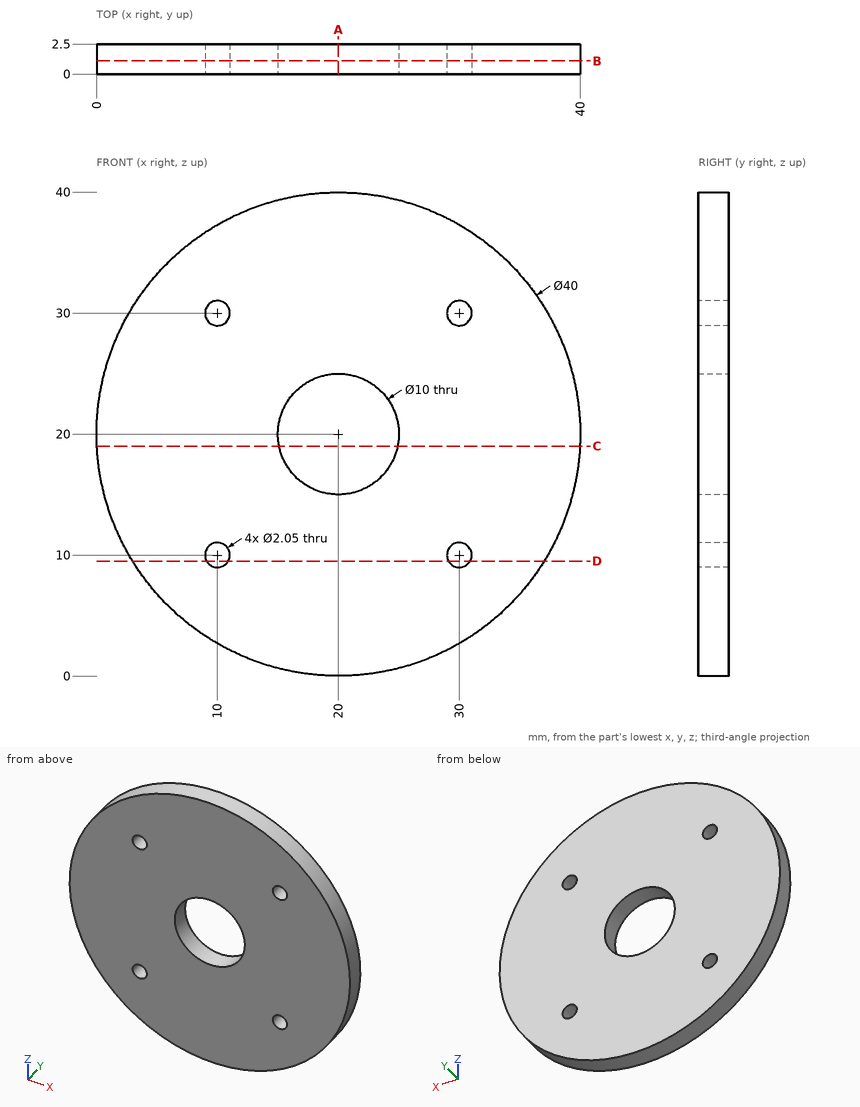
Input: dimensioned drawing with shaded views. Units: mm. Origin: part minimum x, y, z. Coordinates: 2 decimals unless noted, no trailing zeros. Loops run counter-clockwise (first coordinate to the right, second up) from the corner with the lowest first, then second, coordinate; pieces in that order, holes last. Notation, with made-up numbers: (18, 40) -> (65, 40) arc R35 ccw to (65, 79) -> close; hole circle Ø1 at (48.25, -21). An arc over 180 degrees is marked (long way). One line per item, written item: value. Start each with the question number.
Q1. Section query A-A, the plane x = 20. Return the cut outline in (y, z).
Q2. Section query C-C, the plane z = 19. Return the cut outline in (x, y).
Q3. Section query B-B, the plane y = 1.1. Return the cut outline in (x, z) (3 decimals), and give its area (3 significant figures).
Q4. Line query: line 1 along X through (y, z) = (1.85, 10) (1 decimal); line 2 along Z through (x, y) = (17.5, 1.75). Output: solid intervals per line, ascending.
Q5. Contact query for flat-ended pins moving along their axis: P1, Ø2.5, axis at x = 10, z = 10, coming from the -Y side; P2, Ø9, axis at x = 20, z = 20, coming from the +Y side; P3, Ø1, axis at y = 0.5, z = 31, coming from the +X side; P4, Ø1.5, axis at y = 1.5, z = 33.5, coming from the +X side. Output: stop coordinate, or through.
Q6. Section query D-D, the plane z = 9.5. Return the cut outline in (x, y), and give its area (3 significant figures).
Results:
1. outline: (0, 0) -> (2.5, 0) -> (2.5, 15) -> (0, 15) -> close; (0, 25) -> (2.5, 25) -> (2.5, 40) -> (0, 40) -> close
2. outline: (0.03, 0) -> (15.1, 0) -> (15.1, 2.5) -> (0.03, 2.5) -> close; (24.9, 0) -> (39.97, 0) -> (39.97, 2.5) -> (24.9, 2.5) -> close
3. outline: circle Ø40 at (20, 20); hole circle Ø2.05 at (10, 10); hole circle Ø2.05 at (10, 30); hole circle Ø10 at (20, 20); hole circle Ø2.05 at (30, 10); hole circle Ø2.05 at (30, 30)
3. area: 1,160 mm^2
4. line 1: 2.7 to 9, 11 to 29, 31 to 37.3
4. line 2: 0.16 to 15.67, 24.33 to 39.84
5. P1: y = 0
5. P2: through
5. P3: x = 37.02
5. P4: x = 35.41
6. outline: (2.98, 0) -> (9.11, 0) -> (9.11, 2.5) -> (2.98, 2.5) -> close; (10.89, 0) -> (29.11, 0) -> (29.11, 2.5) -> (10.89, 2.5) -> close; (30.89, 0) -> (37.02, 0) -> (37.02, 2.5) -> (30.89, 2.5) -> close
6. area: 76.2 mm^2
